Autodesk Inventor part; units mm, degrees
ref_plane "YZ Plane" through (0, 0, 0) normal (1, 0, 0) x (0, 1, 0)
ref_plane "XZ Plane" through (0, 0, 0) normal (0, 1, 0) x (-1, 0, 0)
ref_plane "XY Plane" through (0, 0, 0) normal (0, 0, 1) x (1, 0, 0)
sketch "Эскиз1" plane through (0, 0, 0) normal (0, 1, 0) x (-1, 0, 0)
  line L0 (14, -5) -> (-14, -5)
  line L1 (-14, -5) -> (-14, 5)
  line L2 (-14, 5) -> (14, 5)
  line L3 (14, 5) -> (14, -5)
  line L4 (-14, -5) -> (14, 5) construction
  line L5 (14, -5) -> (-14, 5) construction
  line L6 (-12, -3) -> (12, -3)
  line L7 (12, -3) -> (12, 3)
  line L8 (12, 3) -> (-12, 3)
  line L9 (-12, 3) -> (-12, -3)
  point P0 (0, 0)
  point P1 (0, 0)
  dimension "d0" = 28
  dimension "d1" = 10
  dimension "d2" = 2
extrude "Выдавливание1" add sketch "Эскиз1" along normal blind 74.2
sketch "Эскиз3" plane through (14, 0, -5) normal (0, 0, -1) x (-1, 0, 0)
  line L0 (0, 0) -> (0, 74.2)
  line L1 (28, 0) -> (28, 74.2)
  line L2 (28, 0) -> (28, 74.2)
  line L3 (0, 0) -> (0, 74.2)
  line L4 (0, 74.2) -> (28, 74.2)
  arc A0 (2, 64.2) -> (26, 64.2) centre (14, 64.2) ccw
  line L5 (26, 0) -> (26, 74.2)
  line L6 (2, 0) -> (2, 74.2)
  line L7 (26, 0) -> (26, 74.2)
  line L8 (26, 64.2) -> (26, 74.2)
  line L9 (26, 74.2) -> (2, 74.2)
  line L10 (2, 64.2) -> (2, 74.2)
  point P0 (14, 0)
  dimension "d10" = 10
extrude "Выдавливание3" cut sketch "Эскиз3" against normal up to surface (2 mm away)
sketch "Эскиз2" plane through (14, 0, 5) normal (1, 0, 0) x (0, 0, -1)
  line L0 (0, 74.2) -> (10, 74.2) construction
  line L1 (10, 74.2) -> (0, 64.2) construction
  line L2 (0, 0) -> (0, 74.2) construction
  line L3 (0, 74.2) -> (10, 64.2) construction
  line L4 (10, 0) -> (10, 74.2) construction
  line L5 (10, 0) -> (0, 10) construction
  line L6 (0, 0) -> (10, 10) construction
  circle A0 centre (5, 69.2) radius 0.5
  circle A1 centre (5, 5) radius 0.5
  point P0 (5, 0)
  dimension "d5" = 1
  dimension "d6" = 1
hole "Отверстие1" at (14, 69.2, 0) at (14, 5, 0) direction (-1, 0, 0) diameter 1 depth 2 countersink diameter 1.5 countersink angle 90
mirror "Зеркальное отражение1" about plane through (0, 0, 0) normal (1, 0, 0) of "Отверстие1"
properties part number "board-1-new"
CAD build for the part. Positions are in the model's coordinates, mm. A direction names the side the tool comes from. Round coordinates to 2 decimals unless told otherwise and drop trailing zeros. Loops run counter-clockwise (first coordinate to the right, second up) from the corner with the lowest first, then second, coordinate; pieces in that order, holes last.
(1) Cut at A-A (x = 0). Give the cut face in (y, z), plus the area to 3 significant figures.
(2) Which spindle directions (+Z, -Z, +X, -X, +Y, -Y) get a long thin tool onto all of the face, cutting with end or side? Do faces 1 (the flat face through (0.2, 0, 3.4)), 2 (the cylindrical face through (0.264, 52.203, -4.014)), 3 (the flat face through (0, 37, 3)). Say none if no direction does.
(3) Cut at C-C (y = 11.5). Give the cut face in (x, z).
(4) Two-plate mould, pull along X, no slides. Class faces 4 (the flat face through (14, 37, 0)), 5 (the flat face through (12, 37, 0)), 6 (the flat face through (0, 28, -5)): +X half, -X half, draft (parallel to the pull), parting line (faces both ways), or undercut.
(5) Cut at B-B (z = 1.5). Give the cut face in (x, y).
(6) Drop a flat-ended pin along its axis: pin 1 (3 mm diameter, centred on x = -2, z = -2, fed in from +Y). Give the stop position or say it passes through.
(7) Wall check: line 1 along Y through (x, z) = (-12.6, 0); line 2 along Z through (x, y) = (9.25, 18.5); line 3 along X through (y, z) = (19.5, -1). Give the ranges that are in metal, low to high.
Findings below:
1. outline: (0, -5) - (52.2, -5) - (52.2, -3) - (0, -3) - close; (0, 3) - (74.2, 3) - (74.2, 5) - (0, 5) - close
1. area: 253 mm2
2. face 1: +Z, -Z, +X, -X, -Y
2. face 2: -Z, +Y
2. face 3: +Y, -Y
3. outline: (-14, -5) - (14, -5) - (14, 5) - (-14, 5) - close; hole (-12, -3) - (12, -3) - (12, 3) - (-12, 3) - close
4. face 4: +X half
4. face 5: undercut
4. face 6: draft
5. outline: (-14, 0) - (-12, 0) - (-12, 74.2) - (-14, 74.2) - close; (12, 0) - (14, 0) - (14, 74.2) - (12, 74.2) - close
6. pin 1: stops at y = 52.61
7. line 1: y = 0 to 4.5, 5.5 to 68.7, 69.7 to 74.2
7. line 2: z = -5 to -3, 3 to 5
7. line 3: x = -14 to -12, 12 to 14
